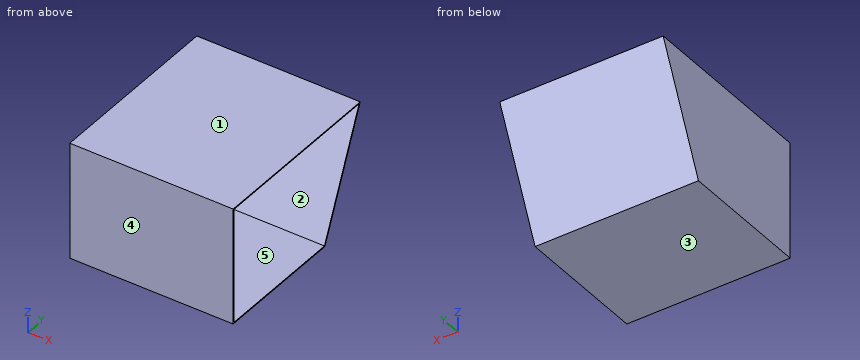
from build123d import *

# Parameters (mm, degrees)
F1_DEPTH = 400
F2_T     = -2.5


with BuildPart() as f1:
    # F0 (on Right) → F1 (new body)
    with BuildSketch(Plane.YZ):
        Polygon((286.688396, 183.30926), (-163.311604, 183.30926), (-163.311604, -101.69074), (161.688396, -101.69074), align=None)
    extrude(amount=-F1_DEPTH)

    # F2
    f2_openings = [f1.faces().sort_by_distance(p)[0] for p in [
        (0, 32.118504, 48.470551),
    ]]
    offset(amount=F2_T, openings=f2_openings)


solid = f1.part
Geometry check sheet. Reference: the model listing, model coordinates, mm. Face numbers are marked on the shaded views. A direction names the side the tool comes from. Give positions to 0.01 mm unless a question says otherwise; leave off trailing zeros. Order: outer loops, then holes, each group sorted by start corner. A loop starts at its lowest first (then second) coordinate and runs counter-clockwise, first axis right, second up.
1. Access from +Z, -Z, +X, -X, +Y, -Y to the whole of each face (thin tool, end or side, straight path). Record for the marked faces 1 and 2.
Completed:
face 1: +Z, +X, -X, +Y, -Y
face 2: +X
2. Sectioned sample at C-C (z = 25). Record the boundary of the cut face in (x, y), then the cut area to 3 significant figures.
Completed:
outline: (-400, -163.31) - (0, -163.31) - (0, -160.81) - (-397.5, -160.81) - (-397.5, 214.52) - (0, 214.52) - (0, 217.25) - (-400, 217.25) - close
area: 3,030 mm2
3. Depth check by flat-ended pin: pin 1 (6 mm diameter, centred on x = -321, y = 237, fed in from -Z); pin 2 (5 mm diameter, centred on x = -279, z = -41.5, fed in from +Y); pin 3 (8 mm diameter, centred on y = -60, z = -16, fed in from +X). Enter the tip coordinate at first touch or a pass-through.
Completed:
pin 1: stops at z = 63.18
pin 2: stops at y = 189.18
pin 3: stops at x = -397.5
4. Sectioned sample at B-B (y = -101). Record the boundary of the cut face in (x, z).
Completed:
outline: (-400, -101.69) - (0, -101.69) - (0, -99.19) - (-397.5, -99.19) - (-397.5, 180.81) - (0, 180.81) - (0, 183.31) - (-400, 183.31) - close
5. Sectioned sample at A-A (x = -334.5). Record the boundary of the cut face in (y, z) (3 decimals).
Completed:
outline: (-163.312, -101.691) - (161.688, -101.691) - (286.688, 183.309) - (-163.312, 183.309) - close; hole (-160.812, -99.191) - (160.055, -99.191) - (282.862, 180.809) - (-160.812, 180.809) - close
6. Draft check along Z on the marked faces 3, 4 and 5. Enter one of: pulls with the +Z half, pulls with the -Z half, needs draft (parallel to the pull), parting line crosses it, or undercut.
Completed:
face 3: pulls with the -Z half
face 4: needs draft
face 5: undercut
7. Scan lines: line 1 (Z direction, x = -43.5, y = 144); line 2 (X direction, y = 177.5, z = 105.5); line 3 (Y direction, x = -179.5, z = 42). Record each from-to range of solid material in increasing order.
Completed:
line 1: z = -101.69 to -99.19, 180.81 to 183.31
line 2: x = -400 to -397.5
line 3: y = -163.31 to -160.81, 221.98 to 224.71
